Input: part model. Units: mm. Frame: model coordinates. Face numbers are marked on the shaded views. A direction names the side the tool comes from. Give positions to 0.01 mm unless a question says otherwise; leave off trailing zeros. Loops run counter-clockwise (first coordinate to the right, second up) from the corner with the lowest first, then second, coordinate; pieces in that order, holes last. Notation, with made-up numbers: M -17,77 L 24,77 A29 cw 24,106 Z; hole C 73.5,58.5 d10. An arc over 180 degrees is marked long. Answer as a JSON object with one key per item and string values. Group by question number.
1) Section query D-D on z = 45.5. Return loops of the section in (x, y), plus the area to 3 significant figures.
2) Access query for the marked faces 1, 2, 3 and 4. Directions: +Z, -Z, +X, -X, +Y, -Y. A direction counts if a zero-diameter tool reaches every point of the face in a straight line with its end or side. Return the directions, or none.
3) Ray query, L1, parallel to X at y = -24, z = 33; L2, parallel to X at y = -9, z = 8; L3, parallel to X at y = -12, z = 24.5. Return the intervals inside material, ascending.
4) First-contact query: P1, Ø9, axis at x = 40, y = -30, coming from the +Z side; P2, Ø2, axis at x = -35.5, y = -20.5, coming from the -Z side; P3, Ø15, axis at x = -34.5, y = -24.5, coming from the +Z side; P4, Ø15, axis at x = -32, z = 21, coming from the -Y side. Flat tips, straight axial feed; report the tip coordinate or a pass-through.
5) Section query C-C on y = -33. Return loops of the section in (x, z).
6) Section query B-B on x = -24. Return loops of the section in (y, z).
7) Section query A-A on z = 13.5. Return loops of the section in (x, y), plus the area to 3 significant figures.
8) Draft query along X for the marked faces 5, 6, 7 and 8. Return one class per face: +X half, -X half, draft (parallel to the pull), parting line (faces both ways), or undercut.
from build123d import *

# Parameters (mm, degrees)
F1_DEPTH = 50
F2_W     = 30
F2_H     = 40
F2_H_2   = 35
F3_DEPTH = 10


with BuildPart() as f1:
    # F0 (on Front) → F1 (new body)
    with BuildSketch(Plane.XZ):
        Polygon((-17.5, 50), (-17.5, 10), (-47.5, 10), (-47.5, 0), (-7.5, 0), (-7.5, 20), (7.5, 20), (7.5, 0), (52.5, 0), (52.5, 15), (22.5, 15), (22.5, 50), (7.5, 50), (7.5, 30), (-7.5, 30), (-7.5, 50), align=None)
    extrude(amount=F1_DEPTH)

    # F2 (on Front) → F3 (join)
    with BuildSketch(Plane.XZ):
        with Locations((-32.5, 30)):
            Rectangle(F2_W, F2_H)
        with Locations((37.5, 32.5)):
            Rectangle(F2_W, F2_H_2)
    extrude(amount=F3_DEPTH)


solid = f1.part
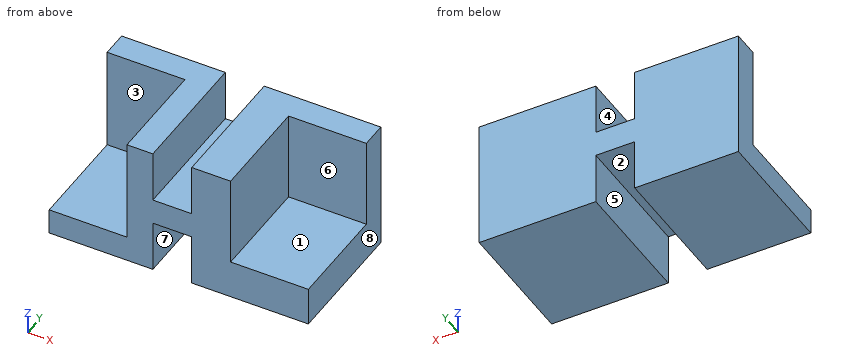
Output:
{
 "1": {"outline": "M -47.5,-10 L -17.5,-10 L -17.5,-50 L -7.5,-50 L -7.5,0 L -47.5,0 Z; M 7.5,-50 L 22.5,-50 L 22.5,-10 L 52.5,-10 L 52.5,0 L 7.5,0 Z", "area": "1,850 mm^2"},
 "2": {"face 1": "+Z, +X, -Y", "face 2": "-Z, +Y, -Y", "face 3": "+Z, -X, -Y", "face 4": "+Z, +Y, -Y"},
 "3": {"L1": "x = -17.5 to -7.5, 7.5 to 22.5", "L2": "x = -47.5 to -7.5, 7.5 to 52.5", "L3": "x = -17.5 to 22.5"},
 "4": {"P1": "stops at z = 15", "P2": "stops at z = 0", "P3": "stops at z = 10", "P4": "stops at y = -10"},
 "5": {"outline": "M -47.5,0 L -7.5,0 L -7.5,20 L 7.5,20 L 7.5,0 L 52.5,0 L 52.5,15 L 22.5,15 L 22.5,50 L 7.5,50 L 7.5,30 L -7.5,30 L -7.5,50 L -17.5,50 L -17.5,10 L -47.5,10 Z"},
 "6": {"outline": "M -50,0 L 0,0 L 0,50 L -10,50 L -10,10 L -50,10 Z"},
 "7": {"outline": "M -47.5,-10 L -17.5,-10 L -17.5,-50 L -7.5,-50 L -7.5,0 L -47.5,0 Z; M 7.5,-50 L 52.5,-50 L 52.5,0 L 7.5,0 Z", "area": "3,050 mm^2"},
 "8": {"face 5": "undercut", "face 6": "draft", "face 7": "undercut", "face 8": "+X half"}
}
